Input: part model. Units: mm. Frame: model coordinates. Give positions to 0.01 mm unless a question says otherwise; leave off trailing zeros. Loops run counter-clockwise (first coordinate to the right, second up) from the corner with the lowest first, then second, coordinate; pieces in that order, holes last. Notation, with made-up numbers: M 29,87.5 L 82,87.5 A22 ccw 82,120.5 Z; hole C 88,-40 d3. An arc over 180 degrees is marked long. One line per item, written item: value. Start each with the question number.
(1) Section C-C on x = 40. Output: boundary loops of the cut face in (y, z).
(2) Section B-B on y = -22. Output: boundary loops of the cut face in (x, z).
(3) Pull-direction query (X, two-part tool) for faces 1 (the cylindrical face through (-41.25, 20.85, 1.97)), 2 (the flat face through (1, 28, 2)), 3 (the cylindrical face through (0.53, 9.02, 1.97)), 4 (the flat face through (-46, 0, 2)); classes: released by +X, released by -X, zero draft, split by the parting line, or undercut.
(4) Section D-D on y = 0. Output: boundary loops of the cut face in (x, z).
(5) Pin query (flat end, axial travel): P1, Ø1.8, axis at x = 8, y = 0, coming from the -Z side. Return the tip coordinate at first contact, or that it passes through.
(6) Section A-A on x = 8. Output: boundary loops of the cut face in (y, z), plus the area to 3 significant figures.
(7) Ray query, line 1 along Y through (x, z) = (0, 1.65); line 2 along Y through (x, z) = (-40, 2.95); line 3 along X through (y, z) = (-23, 2.05). Return the intervals inside material, ascending. Write a range as from..to.
Solid Edge part; units mm, degrees
sketch "Sketch1" plane through (0, 0, 0) normal (0, 0, 1) x (1, 0, 0)
  line L0 (-46, -28) -> (46, -28)
  line L1 (46, -28) -> (46, 28)
  line L2 (46, 28) -> (-46, 28)
  line L3 (-46, 28) -> (-46, -28)
  circle A0 centre (0, 0) radius 4.5
  circle A1 centre (8, 0) radius 1.15
  circle A2 centre (0, 8) radius 1.15
  circle A3 centre (-8, 0) radius 1.15
  circle A4 centre (0, -8) radius 1.15
  circle A5 centre (-40, -22) radius 1.7
  circle A6 centre (-40, 22) radius 1.7
  circle A7 centre (40, -22) radius 1.7
  circle A8 centre (40, 22) radius 1.7
extrude "Protrusion1" add sketch "Sketch1" along normal blind 4
Output values:
1. outline: M -28,0 L -23.7,0 L -23.7,4 L -28,4 Z; M -20.3,0 L 20.3,0 L 20.3,4 L -20.3,4 Z; M 23.7,0 L 28,0 L 28,4 L 23.7,4 Z
2. outline: M -46,0 L -41.7,0 L -41.7,4 L -46,4 Z; M -38.3,0 L 38.3,0 L 38.3,4 L -38.3,4 Z; M 41.7,0 L 46,0 L 46,4 L 41.7,4 Z
3. face 1: undercut
3. face 2: zero draft
3. face 3: undercut
3. face 4: released by -X
4. outline: M -46,0 L -9.15,0 L -9.15,4 L -46,4 Z; M -6.85,0 L -4.5,0 L -4.5,4 L -6.85,4 Z; M 4.5,0 L 6.85,0 L 6.85,4 L 4.5,4 Z; M 9.15,0 L 46,0 L 46,4 L 9.15,4 Z
5. P1: passes through
6. outline: M -28,0 L -1.15,0 L -1.15,4 L -28,4 Z; M 1.15,0 L 28,0 L 28,4 L 1.15,4 Z
6. area: 215 mm²
7. line 1: y = -28..-9.15, -6.85..-4.5, 4.5..6.85, 9.15..28
7. line 2: y = -28..-23.7, -20.3..20.3, 23.7..28
7. line 3: x = -46..-41.37, -38.63..38.63, 41.37..46
